Input: part model. Units: mm. Frame: model coordinates. A direction names the side the tool comes from. Round coordinates to 2 decimals unless told otherwise and drop trailing zeros. Loops run counter-clockwise (first coordinate to the right, second up) from the corner with the lowest first, then second, coordinate; pieces in that order, holes last. Notation, with made-up numbers: (80.25, 62) - (116.25, 62) arc R22 ccw to (116.25, 95) - close; hole circle Ø7 at (-8, -8.5). An arc over 180 degrees is marked (long way). One line per question, with ' | ' between items. Start each with the question number.
from build123d import *

# Parameters (mm, degrees)
CUT_EXTRUDE1_START = -2
CUT_EXTRUDE1_DEPTH = 2
SKETCH4_R          = 1.732050808
CUT_EXTRUDE2_DEPTH = 0.5
CUT_EXTRUDE2_TAPER = 45


with BuildPart() as part:
    # Sketch2 → Revolve1 (revolve)
    with BuildSketch(Plane(origin=(0, 0, 0), x_dir=(0, 0, -1), z_dir=(1, 0, 0))):
        Polygon((-7.8, 3.5), (-4.2, 3.5), (-4, 3.3), (-4, 2), (7.3, 2), (8, 1.3), (8, 0), (-8, 0), (-8, 3.3), align=None)
    revolve(axis=Axis((0, 0, -8), (0, 0, 1)))

    # Sketch3 → Cut-Extrude1 (cut)
    with BuildSketch(Plane.XY.offset(8).offset(CUT_EXTRUDE1_START)):
        Polygon((0, 1.732050808), (-1.5, 0.866025404), (-1.5, -0.866025404), (0, -1.732050808), (1.5, -0.866025404), (1.5, 0.866025404), align=None)
    extrude(amount=CUT_EXTRUDE1_DEPTH, mode=Mode.SUBTRACT)

    # Sketch4 → Cut-Extrude2 (cut)
    with BuildSketch(Plane.XY.offset(8)):
        Circle(SKETCH4_R)
    extrude(amount=-CUT_EXTRUDE2_DEPTH, taper=CUT_EXTRUDE2_TAPER, mode=Mode.SUBTRACT)


solid = part.part
(1) Section B-B, the plane z = -6. Output: boundary loops of the cut face in (x, y), plus the area to 3 significant figures.
(2) Line query: line 1 along Z through (x, y) = (-1.25, 2.25); line 2 along Z through (x, y) = (0.5, -0.5); line 3 along Y through (x, z) = (-1.25, -2). Output: solid intervals per line, ascending. Write a range as from..to.
(3) Reachability of faces 4 (the face through (2.2, 0, 4)), 5 (the face through (0, 0, -8)), 6 (the face through (-1.5, 0, 7)) from +Z, -Z, +X, -X, +Y, -Y: full face, straight path, thin tool, end or side. Return the list, or none.
(4) Pull-direction query (X, two-part tool) for faces 1 (the face through (1.5, 0, 7)), 2 (the face through (2, 0, -2)), 3 (the face through (1.4, -1.4, 8)); classes: released by +X, released by -X, zero draft, split by the parting line, or undercut.
(5) Pin query (flat end, axial travel): P1, Ø2, axis at x = 2, y = -2, coming from the -Z side; P2, Ø1, axis at y = 1.5, z = 0, coming from the -X side. Return the tip coordinate at first contact, or that it passes through.
(6) Section A-A, the plane y = 0. Output: boundary loops of the cut face in (x, z).
Derived:
1) outline: circle Ø4 at (0, 0) | area: 12.6 mm²
2) line 1: z = 4..8 | line 2: z = -8..6 | line 3: y = -1.56..1.56
3) face 4: -Z | face 5: -Z, +X, -X, +Y, -Y | face 6: +Z
4) face 1: undercut | face 2: split by the parting line | face 3: zero draft
5) P1: stops at z = -7.47 | P2: stops at x = -1.73
6) outline: (-3.5, 4.2) - (-3.3, 4) - (-2, 4) - (-2, -7.3) - (-1.3, -8) - (1.3, -8) - (2, -7.3) - (2, 4) - (3.3, 4) - (3.5, 4.2) - (3.5, 7.8) - (3.3, 8) - (1.73, 8) - (1.5, 7.77) - (1.5, 6) - (-1.5, 6) - (-1.5, 7.77) - (-1.73, 8) - (-3.3, 8) - (-3.5, 7.8) - close
